Autodesk Inventor part; units mm, degrees
ref_plane "YZ Plane" through (0, 0, 0) normal (1, 0, 0) x (0, 1, 0)
ref_plane "XZ Plane" through (0, 0, 0) normal (0, 1, 0) x (-1, 0, 0)
ref_plane "XY Plane" through (0, 0, 0) normal (0, 0, 1) x (1, 0, 0)
sketch "Sketch1" plane through (0, 0, 0) normal (0, 0, 1) x (1, 0, 0)
  line L0 (7.5, 25) -> (-7.5, 25) construction
  line L1 (-7.5, 25) -> (-7.5, -25) construction
  line L2 (-7.5, -25) -> (7.5, -25) construction
  line L3 (7.5, -25) -> (7.5, 25) construction
  circle A0 centre (13.75, 3.4269) radius 1.35
  circle A1 centre (-13.75, 3.4269) radius 1.35
  line L4 (20, 13.4269) -> (-20, 13.4269) construction
  line L5 (-20, 13.4269) -> (-20, -6.5731) construction
  line L6 (-20, -6.5731) -> (20, -6.5731) construction
  line L7 (20, -6.5731) -> (20, 13.4269) construction
  line L8 (20, -16.5731) -> (-20, -16.5731)
  line L9 (-20, -16.5731) -> (-20, 23.4269)
  line L10 (-20, 23.4269) -> (20, 23.4269)
  line L11 (20, 23.4269) -> (20, -16.5731)
  line L12 (-20, 3.4269) -> (20, 3.4269) construction
  circle A2 centre (13.75, 18.4269) radius 1.35
  circle A3 centre (-13.75, 18.4269) radius 1.35
  circle A4 centre (-13.75, -11.5731) radius 1.35
  circle A5 centre (13.75, -11.5731) radius 1.35
  point P0 (0, 0)
  dimension "d0" = 20
  dimension "d1" = 40
extrude "Extrusion1" add sketch "Sketch1" along normal blind 3
equation "\"d1\" = 2 * d0"
Geometry check sheet. Reference: the model listing, model coordinates, mm. Coordinates: 2 decimals unless noted, no trailing zeros. Order: outer loops, then holes, each group sorted by start corner. A loop starts at its lowest first (then second) coordinate and runs counter-clockwise, first axis right, second up. Notation, with made-up numbers: M -0.5,-33 L 54.5,-33 A8 ccw 54.5,-29 Z; hole C 38,81 d6. An arc over 180 degrees is marked long. Answer as a JSON object with one key per item and string values.
Q1. Cross-section at B-B on z = 0.5. Record the cut outline in (x, y).
Results are:
{"outline": "M -20,-16.57 L 20,-16.57 L 20,23.43 L -20,23.43 Z; hole C -13.75,-11.57 d2.7; hole C -13.75,3.43 d2.7; hole C -13.75,18.43 d2.7; hole C 13.75,-11.57 d2.7; hole C 13.75,3.43 d2.7; hole C 13.75,18.43 d2.7"}
Q2. Cross-section at A-A on x = -13.75. Record the cut outline in (y, z), and give its area (3 significant figures).
Results are:
{"outline": "M -16.57,0 L -12.92,0 L -12.92,3 L -16.57,3 Z; M -10.22,0 L 2.08,0 L 2.08,3 L -10.22,3 Z; M 4.78,0 L 17.08,0 L 17.08,3 L 4.78,3 Z; M 19.78,0 L 23.43,0 L 23.43,3 L 19.78,3 Z", "area": "95.7 mm²"}
Q3. Release check for a two-part mould opening along Y. For faces 1 (the cylindrical face through (13.457, 19.745, 1.479)), 2 (the flat face through (0, 4, 3)), 3 (the flat face through (0, -16.573, 1)) record: released by +Y, released by -Y, zero draft, split by the parting line, or undercut.
Results are:
{"face 1": "undercut", "face 2": "zero draft", "face 3": "released by -Y"}
Q4. Depth check by flat-ended pin: pin 1 Ø3.5 at (x, y) = (-13.75, 3.43) entering from -Z; pin 2 Ø2.5 at (x, y) = (13.75, 18.43) entering from -Z. Enter the tip coordinate at first touch or a pass-through.
Results are:
{"pin 1": "stops at z = 0", "pin 2": "passes through"}
Q5. Scan lines: line 1 (Y direction, x = -13.75, z = 2.2); line 2 (X direction, y = 18.5, z = 0.45); line 3 (X direction, y = -10.5, z = 0.55). Record each from-to range of solid material in increasing order.
Results are:
{"line 1": "y = -16.57 to -12.92, -10.22 to 2.08, 4.78 to 17.08, 19.78 to 23.43", "line 2": "x = -20 to -15.1, -12.4 to 12.4, 15.1 to 20", "line 3": "x = -20 to -14.57, -12.93 to 12.93, 14.57 to 20"}
